Model file for the job. Use its own axes, mm. Give positions to 0.01 mm unless a question says otherwise; leave off trailing zeros. Order: outer loops, then holes, each group sorted by start corner. A loop starts at its lowest first (then second) coordinate and runs counter-clockwise, first axis right, second up. Notation, with made-up numbers: M 48,-38 L 71,-38 A18 cw 71,-16 Z; hole C -1,50.5 d10. An arc over 180 degrees is marked long. Return JSON: item names as keys, results as strings. Group by question number.
1. Slice it at A-A on x = 32. List the corners of the cut face in (y, z), then the cut area to 3 significant figures.
2. Slice it at B-B on z = -0.6. List the corners of the cut face in (x, y), then the cut area to 3 significant figures.
3. Wall check: probe 1 along Y at (x, z) = (-16, -0.55); probe 2 along Y at (x, z) = (42, -0.5); probe 3 along X at (y, z) = (29.5, -0.35). Give the ranges that are in metal, low to high. Write a range as [from, to].
4. Pin check, flat tip, straight feed: pin 1 (5 mm diameter, centred on x = -35, y = 23.5, fed in from -Z). Stop position of the tip, or through.
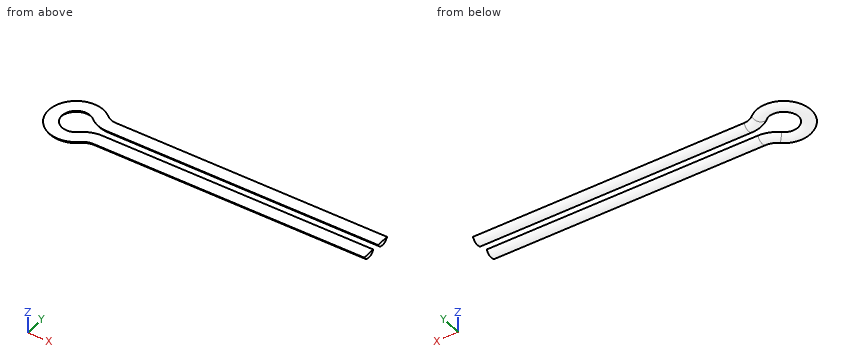
from build123d import *


with BuildPart() as f3:
    # F3: sweep along a path in F0
    with BuildLine(Plane.XY) as f3_path:
        Line((67.8468741477, 27.1481485665), (-27.0727876186, 27.1481485665))
        ThreePointArc((-27.0727876186, 27.1481485665), (-30.6083215245, 27.7940050995), (-33.6871658963, 29.6481485665))
        ThreePointArc((-33.6871658963, 29.6481485665), (-41.9943550351, 25.8981485665), (-33.6871658963, 22.1481485665))
        ThreePointArc((-33.6871658963, 22.1481485665), (-30.6083215245, 24.0022920334), (-27.0727876186, 24.6481485665))
        Line((-27.0727876186, 24.6481485665), (67.8468741477, 24.6481485665))
    # F2 (on plane+point) → F3 (sweep)
    with BuildSketch(Plane.YZ.offset(67.8468741477)):
        with BuildLine():
            Line((24.6481485665, 0), (20.0226833864, 0))
            ThreePointArc((20.0226833864, 0), (22.3354159764, -1.5506486599), (24.6481485665, 0))
        make_face()
    sweep(path=f3_path.line)


solid = f3.part
Result:
{
 "1": {"outline": "M 20.02,0 A2.5 ccw 24.65,0 Z; M 27.15,0 A2.5 ccw 31.77,0 Z", "area": "10.4 mm2"},
 "2": {"outline": "M -33.46,21.89 A5.35 cw long -33.46,29.91 A9.65 ccw -27.07,27.5 L 67.85,27.5 L 67.85,31.42 L -27.07,31.42 A5.73 cw -30.86,32.85 A9.27 ccw long -30.86,18.94 A5.73 cw -27.07,20.37 L 67.85,20.37 L 67.85,24.3 L -27.07,24.3 A9.65 ccw Z", "area": "920 mm2"},
 "3": {"probe 1": "y = [20.33, 24.34], [27.46, 31.46]", "probe 2": "y = [20.3, 24.37], [27.42, 31.5]", "probe 3": "x = [-45.73, -40.71], [-33.24, 67.85]"},
 "4": {"pin 1": "stops at z = -0.89"}
}
